Work out the finished part from the listing and answer in its coordinate system (mm). A direction names the side the tool comes from. Give positions to 0.01 mm unless a question says otherwise; leave off trailing zeros. Order: outer loops, then holes, each group sorted by start corner. A loop starts at its lowest first (then second) coordinate and runs counter-clockwise, first axis right, second up.
```python
from build123d import *

# Parameters (mm, degrees)
F0_W     = 1200
F0_H     = 800
F0_W_2   = 1040
F0_H_2   = 250
F1_DEPTH = 15
F2_W     = 185.065291822
F2_H     = 140
F3_DEPTH = 40
F2_W_2   = 100
F2_H_2   = 80
F2_W_3   = 116.4537014898
F2_H_3   = 141.4459940791
F2_W_4   = 112.9816351
F2_W_5   = 102.8472425875
F2_W_6   = 112.1940789286
F2_W_7   = 183.0065995455
F4_DEPTH = 40


with BuildPart() as f1:
    # F0 (on Front) → F1 (new body)
    with BuildSketch(Plane.XZ):
        with Locations((-16.7594370905, 0)):
            Rectangle(F0_W, F0_H)
        with Locations((-16.7594370905, -195)):
            Rectangle(F0_W_2, F0_H_2, mode=Mode.SUBTRACT)
        with Locations((-16.7594370905, 195)):
            Rectangle(F0_W_2, F0_H_2, mode=Mode.SUBTRACT)
    extrude(amount=F1_DEPTH)

    # F2 (on face) → F3 (join)
    with BuildSketch(Plane(origin=(0, 0, 0), x_dir=(-1, 0, 0), z_dir=(0, 1, 0))):
        with Locations((20.5517672002, 0)):
            Rectangle(F2_W, F2_H)
        Polygon((616.7594370905, -70), (616.7594370905, 70), (536.7594370905, 70), (503.7778019905, 70), (503.7778019905, -70), (536.7594370905, -70), align=None)
        Polygon((616.7594370905, -400), (616.7594370905, -320), (536.7594370905, -320), (504.5653581619, -320), (504.5653581619, -400), align=None)
        Polygon((-503.2405629095, -320), (-583.2405629095, -320), (-583.2405629095, -400), (-480.393320322, -400), (-480.393320322, -320), align=None)
        Polygon((-503.2405629095, 70), (-503.2405629095, 71.4459940791), (-583.2405629095, 71.4459940791), (-583.2405629095, -70), (-503.2405629095, -70), (-466.7868614197, -70), (-466.7868614197, 70), align=None)
        Polygon((-483.2405629095, 320), (-483.2405629095, 400), (-583.2405629095, 400), (-583.2405629095, 320), (-503.2405629095, 320), align=None)
        Polygon((616.7594370905, 400), (516.7594370905, 400), (516.7594370905, 320), (536.7594370905, 320), (616.7594370905, 320), align=None)
    extrude(amount=F3_DEPTH)

    # F2 (on face) → F4 (join)
    with BuildSketch(Plane(origin=(0, 0, 0), x_dir=(-1, 0, 0), z_dir=(0, 1, 0))):
        with Locations((566.7594370905, 360)):
            Rectangle(F2_W_2, F2_H_2)
        with Locations((-533.2405629095, 360)):
            Rectangle(F2_W_2, F2_H_2)
        with Locations((-525.0137121646, 0.7229970396)):
            Rectangle(F2_W_3, F2_H_3)
        with Locations((560.2686195405, 0)):
            Rectangle(F2_W_4, F2_H)
        with Locations((20.5517672002, 0)):
            Rectangle(F2_W, F2_H)
        with Locations((-531.8169416158, -360)):
            Rectangle(F2_W_5, F2_H_2)
        with Locations((560.6623976262, -360)):
            Rectangle(F2_W_6, F2_H_2)
        with Locations((7.9610347748, 360)):
            Rectangle(F2_W_7, F2_H_2)
        with Locations((20.5517672002, -360)):
            Rectangle(F2_W, F2_H_2)
    extrude(amount=F4_DEPTH)

    # F5: F1 across face


with BuildPart() as f1_1:
    add(f1.part)
    add(f1.part.mirror(Plane(origin=(-20.5517672002, 40, 0), x_dir=(-1, 0, 0), z_dir=(0, 1, 0))))


solid = f1_1.part
```
1. The part is cut by section C-C (z = 0). Write down the section's boundary in (x, y), then the cut area to 3 significant figures.
Findings below:
outline: (-616.76, -15) - (583.24, -15) - (583.24, 95) - (-616.76, 95) - close; hole (-503.78, 0) - (-113.08, 0) - (-113.08, 80) - (-503.78, 80) - close; hole (71.98, 0) - (466.79, 0) - (466.79, 80) - (71.98, 80) - close
area: 69,200 mm2
2. Given P1, Ø1.2, axis at x = 492.5, z = 71, coming from the +Y side, flat-ended and moving along its own axis, determine where the tip first touches the part or whether it passes through.
Findings below:
P1: stops at y = 80
3. The mould has two halves that part along X. Classify faces 1 (the face through (-25, -15, 6)), 2 (the face through (-8, 41, 320)), 3 (the face through (583.241, 39, -6)): pulls with the +X half, pulls with the -X half, needs draft (parallel to the pull), parting line crosses it, or undercut.
Findings below:
face 1: needs draft
face 2: undercut
face 3: pulls with the +X half
4. The part is cut by section A-A (z = -238.5). Write down the section's boundary in (x, y).
Findings below:
outline: (-616.76, -15) - (-536.76, -15) - (-536.76, 0) - (-616.76, 0) - close; (-616.76, 80) - (-536.76, 80) - (-536.76, 95) - (-616.76, 95) - close; (503.24, -15) - (583.24, -15) - (583.24, 0) - (503.24, 0) - close; (503.24, 80) - (583.24, 80) - (583.24, 95) - (503.24, 95) - close
5. The part is cut by section B-B (x = -450). Write down the section's boundary in (y, z), then the cut area to 3 significant figures.
Findings below:
outline: (-15, -400) - (0, -400) - (0, -320) - (-15, -320) - close; (-15, -70) - (0, -70) - (0, 70) - (-15, 70) - close; (-15, 320) - (0, 320) - (0, 400) - (-15, 400) - close; (80, -400) - (95, -400) - (95, -320) - (80, -320) - close; (80, -70) - (95, -70) - (95, 70) - (80, 70) - close; (80, 320) - (95, 320) - (95, 400) - (80, 400) - close
area: 9,000 mm2
6. The part is cut by section D-D (y = 32). State how many separate pieces and enclosed holes the cut face has, then the cut area to 3 significant figures.
Findings below:
separate pieces: 9
enclosed holes: 0
area: 121,000 mm2
7. Straight lines are drawn through the part: probe 1 along Z at (x, y) = (-53, 12); probe 2 along X at (y, z) = (21, -26.5); probe 3 along X at (y, z) = (-2.5, 147). For each, find the intervals that lie inside material, in ascending order.
Findings below:
probe 1: z = -400 to -320, -70 to 70, 320 to 400
probe 2: x = -616.76 to -503.78, -113.08 to 71.98, 466.79 to 583.24
probe 3: x = -616.76 to -536.76, 503.24 to 583.24
8. Which of the six approach directions +Z, -Z, +X, -X, +Y, -Y give full straight-line access (tool end or side, diameter ignored) to faces 4 (the face through (-8, 41, -70)), 5 (the face through (-312, 0, -359)), 6 (the face through (524, 41, 71.446)), 7 (the face through (480.393, 41, -361)), 8 (the face through (-25, 39, 400))?
Findings below:
face 4: none
face 5: +Z, -Z
face 6: +X, -X
face 7: -Z
face 8: +Z, +X, -X, +Y, -Y
